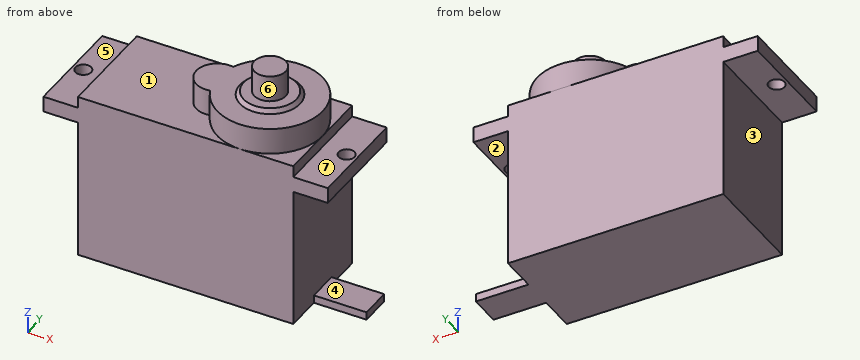
```python
from build123d import *

# Parameters (mm, degrees)
SKETCH3_R           = 3
BOSS_EXTRUDE1_DEPTH = 2.5
SKETCH4_R           = 6
BOSS_EXTRUDE2_DEPTH = 0.7
BOSS_EXTRUDE3_DEPTH = 5
SKETCH6_W           = 40.9
SKETCH6_H           = 20
BOSS_EXTRUDE4_DEPTH = 32
SKETCH7_W           = 3
SKETCH7_H           = 20
BOSS_EXTRUDE5_DEPTH = 20
SKETCH8_OUTSIDE_W   = 101.628
SKETCH8_OUTSIDE_H   = 40.728
SKETCH8_OUTSIDE_W_2 = 54
SKETCH8_OUTSIDE_H_2 = 30
CUT_EXTRUDE1_DEPTH  = 66.626595219
CUT_EXTRUDE2_REACH  = 50.893
SKETCH10_R          = 1.5
SKETCH11_W          = 1.5
SKETCH11_H          = 6
BOSS_EXTRUDE6_DEPTH = 10
CHAMFER1_SIZE       = 1


with BuildPart() as part:
    # Sketch3 → Boss-Extrude1 (new, symmetric)
    with BuildSketch(Plane.XY):
        Circle(SKETCH3_R)
    extrude(amount=BOSS_EXTRUDE1_DEPTH, both=True)

    # Sketch4 → Boss-Extrude2 (add)
    with BuildSketch(Plane(origin=(0, 0, -2.5), x_dir=(-1, 0, 0), z_dir=(0, 0, -1))):
        Circle(SKETCH4_R)
    extrude(amount=BOSS_EXTRUDE2_DEPTH)

    # Sketch5 → Boss-Extrude3 (add)
    with BuildSketch(Plane(origin=(0, 0, -3.2), x_dir=(-1, 0, 0), z_dir=(0, 0, -1))):
        with BuildLine():
            ThreePointArc((9.2, 3.919183588), (-10, 0), (9.2, -3.919183588))
            ThreePointArc((9.2, -3.919183588), (14, 0), (9.2, 3.919183588))
        make_face()
    extrude(amount=BOSS_EXTRUDE3_DEPTH)

    # Sketch6 → Boss-Extrude4 (add)
    with BuildSketch(Plane(origin=(0, 0, -8.2), x_dir=(-1, 0, 0), z_dir=(0, 0, -1))):
        with Locations((10.45, 0)):
            Rectangle(SKETCH6_W, SKETCH6_H)
    extrude(amount=BOSS_EXTRUDE4_DEPTH)

    # Sketch7 → Boss-Extrude5 (add)
    with BuildSketch(Plane(origin=(10, 0, 0), x_dir=(0, 0, -1), z_dir=(1, 0, 0))):
        with Locations((11.9, 0)):
            Rectangle(SKETCH7_W, SKETCH7_H)
    boss_extrude5 = extrude(amount=BOSS_EXTRUDE5_DEPTH)

    # Mirror1: Boss-Extrude5 across plane
    add(boss_extrude5.mirror(Plane(origin=(-10.45, 0, 0), x_dir=(0, 0, 1), z_dir=(1, 0, 0))))

    # Sketch8 outside → Cut-Extrude1 (cut, through all)
    with BuildSketch(Plane.XY):
        with Locations((-10.45, 0)):
            Rectangle(SKETCH8_OUTSIDE_W, SKETCH8_OUTSIDE_H)
        with Locations((-10.45, 0)):
            Rectangle(SKETCH8_OUTSIDE_W_2, SKETCH8_OUTSIDE_H_2, mode=Mode.SUBTRACT)
    extrude(amount=-CUT_EXTRUDE1_DEPTH, mode=Mode.SUBTRACT)

    # Sketch10 → Cut-Extrude2 (cut, up to next)
    with BuildSketch(Plane.XY.offset(-10.4), mode=Mode.PRIVATE) as cut_extrude2_sk1:
        with Locations((-35.45, 0)):
            Circle(SKETCH10_R)
    cut_extrude2_tool1 = extrude(cut_extrude2_sk1.sketch, amount=-CUT_EXTRUDE2_REACH, mode=Mode.PRIVATE) & part.part
    # Sketch10 → Cut-Extrude2 (cut, up to next)
    with BuildSketch(Plane.XY.offset(-10.4), mode=Mode.PRIVATE) as cut_extrude2_sk2:
        with Locations(Location((14.55, 0, 0), (0, 0, 270))):
            Circle(SKETCH10_R)
    cut_extrude2_tool2 = extrude(cut_extrude2_sk2.sketch, amount=-CUT_EXTRUDE2_REACH, mode=Mode.PRIVATE) & part.part
    add(cut_extrude2_tool1.solids().sort_by_distance((-35.45, 0, -10.4))[0], mode=Mode.SUBTRACT)
    add(cut_extrude2_tool2.solids().sort_by_distance((14.55, 0, -10.4))[0], mode=Mode.SUBTRACT)

    # Sketch11 → Boss-Extrude6 (add)
    with BuildSketch(Plane(origin=(10, 0, 0), x_dir=(0, 0, -1), z_dir=(1, 0, 0))):
        with Locations((39.45, 0)):
            Rectangle(SKETCH11_W, SKETCH11_H)
    extrude(amount=BOSS_EXTRUDE6_DEPTH)

    # Chamfer1
    # the kernel refuses this chamfer: 1 mm, written as the material it takes off along each edge
    with BuildSketch(Plane(origin=(0, 0, -2.5), x_dir=(-1, 0, 0), z_dir=(0, -1, 0))) as chamfer1_piece_1_section:
        Polygon((6, CHAMFER1_SIZE), (6 - CHAMFER1_SIZE, 0), (6, 0), align=None)
    chamfer1_piece_1 = revolve(axis=Axis((0, 0, -2.5), (0, 0, -1)), mode=Mode.PRIVATE)
    chamfer1_piece_1 = split(chamfer1_piece_1, bisect_by=Plane(origin=(5.354214233, 0, -3.2), z_dir=(0, 0, 1)), keep=Keep.TOP, mode=Mode.PRIVATE)
    add(chamfer1_piece_1, mode=Mode.SUBTRACT)


solid = part.part
```
Check sheet for the modelled part. Datum: model origin and axes. Units: mm. Face numbers are marked on the shaded views. A direction names the side the tool comes from. Round coordinates to 2 decimals unless told otherwise and drop trailing zeros. Loops run counter-clockwise (first coordinate to the right, second up) from the corner with the lowest first, then second, coordinate; pieces in that order, holes last. Notation, with made-up numbers: (-19.75, 48.25) -> (11.25, 48.25) arc R7 ccw to (11.25, 55.25) -> close; hole circle Ø4 at (53.25, 49.5). An arc over 180 degrees is marked (long way). Write item = value, one per line. Start each with the question number.
1) Thickness scan on probe 1 along Z at (x, y) = (11.5, 1.25); probe 2 along Z at (x, y) = (-32.5, 1); probe 3 along Z at (x, y) = (14, 1). Record the ranges inside material, lowest first.
2) Release check for a two-part mould opening along Z. For the marked faces 1, 2 and 3 record: released by +Z, released by -Z, zero draft, split by the parting line, or undercut.
3) Sectioned sample at D-D, the plane y = -6.5. Record the cut outline in (x, z).
4) Sectioned sample at A-A, the plane x = -35.45. Record the cut outline in (y, z), plus the area to 3 significant figures.
5) Set-up check for the marked faces 4, 5, 6 and 7: record each of +Z, -Z, +X, -X, +Y, -Y from which the full face is reachable in a straight line by a thin tool's end or side.
6) Sectioned sample at C-C, the plane z = -11.5. Record the cut outline in (x, y), plus the area to 3 significant figures.
7) Sectioned sample at B-B, the plane x = -10. Record the cut outline in (y, z).
8) Gauge pin test, flat ends, axial feed: pin 1 Ø8 at (x, z) = (11.5, -2) entering from +Y; pin 2 Ø0.7 at (y, z) = (0, -9.5) entering from -X; pin 3 Ø2.5 at (x, y) = (-35.45, 0) entering from -Z; pin 4 Ø4 at (x, y) = (-10, 3) entering from +Z. Record the tip position at first contact, or that the pin passes through.
Results are:
q1.probe_1 = -40.2 to -38.7, -13.4 to -10.4
q1.probe_2 = -13.4 to -10.4
q1.probe_3 = -40.2 to -38.7
q2.face_1 = released by +Z
q2.face_2 = undercut
q2.face_3 = zero draft
q3.outline = (-37.45, -13.4) -> (-30.9, -13.4) -> (-30.9, -40.2) -> (10, -40.2) -> (10, -13.4) -> (16.55, -13.4) -> (16.55, -10.4) -> (10, -10.4) -> (10, -8.2) -> (7.6, -8.2) -> (7.6, -3.2) -> (-7.6, -3.2) -> (-7.6, -8.2) -> (-30.9, -8.2) -> (-30.9, -10.4) -> (-37.45, -10.4) -> close
q4.outline = (-10, -13.4) -> (-1.5, -13.4) -> (-1.5, -10.4) -> (-10, -10.4) -> close; (1.5, -13.4) -> (10, -13.4) -> (10, -10.4) -> (1.5, -10.4) -> close
q4.area = 51.0 mm^2
q5.face_4 = +X, +Y, -Y
q5.face_5 = +Z, -X, +Y, -Y
q5.face_6 = +Z
q5.face_7 = +Z, +X, +Y, -Y
q6.outline = (-37.45, -10) -> (16.55, -10) -> (16.55, 10) -> (-37.45, 10) -> close; hole circle Ø3 at (-35.45, 0); hole circle Ø3 at (14.55, 0)
q6.area = 1,070 mm^2
q7.outline = (-10, -40.2) -> (10, -40.2) -> (10, -8.2) -> (4, -8.2) -> (4, -3.2) -> (-4, -3.2) -> (-4, -8.2) -> (-10, -8.2) -> close
q8.pin_1 = 6.4
q8.pin_2 = -30.9
q8.pin_3 = through
q8.pin_4 = -3.2
